The model under review builds one solid part; all positions refer to its coordinate system, in mm. Face numbers are marked on the shaded views. Round coordinates to 2 decimals unless told otherwise and drop trailing zeros. Order: outer loops, then holes, each group sorted by start corner. A loop starts at its lowest first (then second) coordinate and runs counter-clockwise, first axis right, second up.
1) Consider section A-A (x = 0). Give the boundary of the cut face in (y, z).
2) To check wall thickness, follow L1, parallel to X at y = 12.5, z = 0; L2, parallel to Z at x = -7, y = 6.5. State the ranges of each line that lie inside material, in increasing order.
3) Clearance check with flat-ended pins moving along their axes: P1, Ø10, axis at x = 4, y = 25.5, coming from the +Z side; P2, Ø2, axis at x = 7, y = 15, coming from the +Z side; P3, Ø10, axis at x = 10.5, y = 14, coming from the -Z side; P4, Ø8, axis at x = -18, y = 39.5, coming from the -Z side. State where each tip first meets the part, or that it passes through.
4) Mouldability with a two-part tool opening along X and no side actions: class the marked faces 1, 2 and 3 as pulls with the +X half, pulls with the -X half, needs draft (parallel to the pull), parting line crosses it, or undercut.
5) Consider section B-B (z = 0). Give the boundary of the cut face in (x, y).
6) Consider section C-C (y = 11). Give the boundary of the cut face in (x, z).
from build123d import *

# Parameters (mm, degrees)
SKETCH1_R           = 28.2067
BOSS_EXTRUDE1_DEPTH = 33.5788
SHELL1_T            = -4.064


with BuildPart() as part:
    # Sketch1 → Boss-Extrude1 (new body)
    with BuildSketch(Plane(origin=(0, 0, 0), x_dir=(1, 0, 0), z_dir=(0, 1, 0))):
        with Locations(Location((0, 0, 0), (0, 0, 270))):
            Circle(SKETCH1_R)
    extrude(amount=BOSS_EXTRUDE1_DEPTH)

    # Sketch2 → Revolve1 (revolve)
    with BuildSketch(Plane.XY, mode=Mode.PRIVATE) as revolve1_sk:
        with BuildLine():
            Line((0, 33.5788), (-28.2067, 33.5788))
            ThreePointArc((-28.2067, 33.5788), (-16.511981345, 46.121893901), (0, 50.753321445))
            Line((0, 50.753321445), (0, 33.5788))
        make_face()
    revolve(revolve1_sk.sketch.rotate(Axis((0, 50.753321445, 0), (0, -1, 0)), 180), axis=Axis((0, 50.753321445, 0), (0, -1, 0)))

    # Shell1
    shell1_openings = [part.faces().sort_by_distance(p)[0] for p in [
        (0, 0, 0),
    ]]
    offset(amount=SHELL1_T, openings=shell1_openings)


solid = part.part
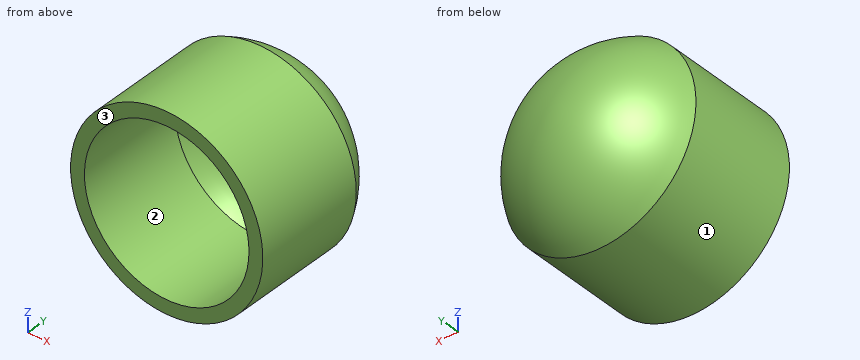
Answer below:
1. outline: (0, -28.21) - (33.58, -28.21) arc R31.75 ccw to (33.58, 28.21) - (0, 28.21) - (0, 24.14) - (32.55, 24.14) arc R27.69 cw to (32.55, -24.14) - (0, -24.14) - close
2. L1: x = -28.21 to -24.14, 24.14 to 28.21
2. L2: z = -27.32 to -23.11, 23.11 to 27.32
3. P1: stops at z = 28.21
3. P2: stops at z = 27.56
3. P3: stops at z = -27.67
3. P4: stops at z = -21.59
4. face 1: parting line crosses it
4. face 2: undercut
4. face 3: needs draft
5. outline: (-28.21, 0) - (-24.14, 0) - (-24.14, 32.55) arc R27.69 cw to (24.14, 32.55) - (24.14, 0) - (28.21, 0) - (28.21, 33.58) arc R31.75 ccw to (-28.21, 33.58) - close
6. outline: circle Ø56.41 at (0, 0); hole circle Ø48.29 at (0, 0)
